Input: part model. Units: mm. Frame: model coordinates. Face numbers are marked on the shaded views. A direction names the side the tool comes from. Give positions to 0.01 mm unless a question says otherwise; leave off trailing zeros. Order: outer loops, then holes, each group sorted by start corner. A loop starts at its lowest first (then second) coordinate and runs counter-clockwise, first axis right, second up. Notation, with made-up numbers: M 40,69 L 72,69 A18 ccw 72,94 Z; hole C -27.5,89 d4. An arc over 180 degrees is marked long. Use a Markdown table: item, result.
from build123d import *

# Parameters (mm, degrees)
SKETCH_1_R      = 5.05
SKETCH_1_R_2    = 4.875
EXTRUDE_1_DEPTH = 10
FILLET_1_R      = 1


with BuildPart() as part:
    # 草图1 → 凸台-拉伸1 (new body)
    with BuildSketch(Plane.XY):
        with BuildLine():
            Line((100.75, 13), (39.610949593, 13))
            ThreePointArc((39.610949593, 13), (42.143955384, 14.911655633), (44.291298968, 17.248204611))
            ThreePointArc((44.291298968, 17.248204611), (43.91314903, 18.189421895), (43.515000291, 19.122355404))
            ThreePointArc((43.515000291, 19.122355404), (39.135260233, 19.155630081), (34.883671922, 18.103381529))
            ThreePointArc((34.883671922, 18.103381529), (34.03604328, 19.65071875), (33.119824259, 21.158455298))
            ThreePointArc((33.119824259, 21.158455298), (36.156892392, 24.314314506), (38.317945706, 28.123917996))
            ThreePointArc((38.317945706, 28.123917996), (37.709075956, 28.935191673), (37.083032847, 29.733287767))
            ThreePointArc((37.083032847, 29.733287767), (32.843916692, 28.631868497), (29.009539705, 26.515082418))
            ThreePointArc((29.009539705, 26.515082418), (27.790312967, 27.790312967), (26.515082418, 29.009539705))
            ThreePointArc((26.515082418, 29.009539705), (28.631868497, 32.843916692), (29.733287767, 37.083032847))
            ThreePointArc((29.733287767, 37.083032847), (28.935191673, 37.709075956), (28.123917996, 38.317945706))
            ThreePointArc((28.123917996, 38.317945706), (24.314314506, 36.156892392), (21.158455298, 33.119824259))
            ThreePointArc((21.158455298, 33.119824259), (19.65071875, 34.03604328), (18.103381529, 34.883671922))
            ThreePointArc((18.103381529, 34.883671922), (19.155630081, 39.135260233), (19.122355404, 43.515000291))
            ThreePointArc((19.122355404, 43.515000291), (18.189421895, 43.91314903), (17.248204611, 44.291298968))
            ThreePointArc((17.248204611, 44.291298968), (14.127731967, 41.217883822), (11.865457128, 37.46750481))
            ThreePointArc((11.865457128, 37.46750481), (10.171960525, 37.962273492), (8.457965105, 38.380539546))
            ThreePointArc((8.457965105, 38.380539546), (8.37396713, 42.759600464), (7.208266121, 46.981492378))
            ThreePointArc((7.208266121, 46.981492378), (6.204073074, 47.124613567), (5.197054586, 47.2462734))
            ThreePointArc((5.197054586, 47.2462734), (2.978367841, 43.469944586), (1.763847663, 39.261836826))
            ThreePointArc((1.763847663, 39.261836826), (0, 39.3014375), (-1.763847663, 39.261836826))
            ThreePointArc((-1.763847663, 39.261836826), (-2.978367841, 43.469944586), (-5.197054586, 47.2462734))
            ThreePointArc((-5.197054586, 47.2462734), (-6.204073074, 47.124613567), (-7.208266121, 46.981492378))
            ThreePointArc((-7.208266121, 46.981492378), (-8.37396713, 42.759600464), (-8.457965105, 38.380539546))
            ThreePointArc((-8.457965105, 38.380539546), (-10.171960525, 37.962273492), (-11.865457128, 37.46750481))
            ThreePointArc((-11.865457128, 37.46750481), (-14.127731967, 41.217883822), (-17.248204611, 44.291298968))
            ThreePointArc((-17.248204611, 44.291298968), (-18.189421895, 43.91314903), (-19.122355404, 43.515000291))
            ThreePointArc((-19.122355404, 43.515000291), (-19.155630081, 39.135260233), (-18.103381529, 34.883671922))
            ThreePointArc((-18.103381529, 34.883671922), (-19.65071875, 34.03604328), (-21.158455298, 33.119824259))
            ThreePointArc((-21.158455298, 33.119824259), (-24.314314506, 36.156892392), (-28.123917996, 38.317945706))
            ThreePointArc((-28.123917996, 38.317945706), (-28.935191673, 37.709075956), (-29.733287767, 37.083032847))
            ThreePointArc((-29.733287767, 37.083032847), (-28.631868497, 32.843916692), (-26.515082418, 29.009539705))
            ThreePointArc((-26.515082418, 29.009539705), (-27.790312967, 27.790312967), (-29.009539705, 26.515082418))
            ThreePointArc((-29.009539705, 26.515082418), (-32.843916692, 28.631868497), (-37.083032847, 29.733287767))
            ThreePointArc((-37.083032847, 29.733287767), (-37.709075956, 28.935191673), (-38.317945706, 28.123917996))
            ThreePointArc((-38.317945706, 28.123917996), (-36.156892392, 24.314314506), (-33.119824259, 21.158455298))
            ThreePointArc((-33.119824259, 21.158455298), (-34.03604328, 19.65071875), (-34.883671922, 18.103381529))
            ThreePointArc((-34.883671922, 18.103381529), (-39.135260233, 19.155630081), (-43.515000291, 19.122355404))
            ThreePointArc((-43.515000291, 19.122355404), (-43.91314903, 18.189421895), (-44.291298968, 17.248204611))
            ThreePointArc((-44.291298968, 17.248204611), (-41.217883822, 14.127731967), (-37.46750481, 11.865457128))
            ThreePointArc((-37.46750481, 11.865457128), (-37.962273492, 10.171960525), (-38.380539546, 8.457965105))
            ThreePointArc((-38.380539546, 8.457965105), (-42.759600464, 8.37396713), (-46.981492378, 7.208266121))
            ThreePointArc((-46.981492378, 7.208266121), (-47.124613567, 6.204073074), (-47.2462734, 5.197054586))
            ThreePointArc((-47.2462734, 5.197054586), (-43.469944586, 2.978367841), (-39.261836826, 1.763847663))
            ThreePointArc((-39.261836826, 1.763847663), (-39.3014375, 0), (-39.261836826, -1.763847663))
            ThreePointArc((-39.261836826, -1.763847663), (-43.469944586, -2.978367841), (-47.2462734, -5.197054586))
            ThreePointArc((-47.2462734, -5.197054586), (-47.124613567, -6.204073074), (-46.981492378, -7.208266121))
            ThreePointArc((-46.981492378, -7.208266121), (-42.759600464, -8.37396713), (-38.380539546, -8.457965105))
            ThreePointArc((-38.380539546, -8.457965105), (-37.962273492, -10.171960525), (-37.46750481, -11.865457128))
            ThreePointArc((-37.46750481, -11.865457128), (-41.217883822, -14.127731967), (-44.291298968, -17.248204611))
            ThreePointArc((-44.291298968, -17.248204611), (-43.91314903, -18.189421895), (-43.515000291, -19.122355404))
            ThreePointArc((-43.515000291, -19.122355404), (-39.135260233, -19.155630081), (-34.883671922, -18.103381529))
            ThreePointArc((-34.883671922, -18.103381529), (-34.03604328, -19.65071875), (-33.119824259, -21.158455298))
            ThreePointArc((-33.119824259, -21.158455298), (-36.156892392, -24.314314506), (-38.317945706, -28.123917996))
            ThreePointArc((-38.317945706, -28.123917996), (-37.709075956, -28.935191673), (-37.083032847, -29.733287767))
            ThreePointArc((-37.083032847, -29.733287767), (-32.843916692, -28.631868497), (-29.009539705, -26.515082418))
            ThreePointArc((-29.009539705, -26.515082418), (-27.790312967, -27.790312967), (-26.515082418, -29.009539705))
            ThreePointArc((-26.515082418, -29.009539705), (-28.631868497, -32.843916692), (-29.733287767, -37.083032847))
            ThreePointArc((-29.733287767, -37.083032847), (-28.935191673, -37.709075956), (-28.123917996, -38.317945706))
            ThreePointArc((-28.123917996, -38.317945706), (-24.314314506, -36.156892392), (-21.158455298, -33.119824259))
            ThreePointArc((-21.158455298, -33.119824259), (-19.65071875, -34.03604328), (-18.103381529, -34.883671922))
            ThreePointArc((-18.103381529, -34.883671922), (-19.155630081, -39.135260233), (-19.122355404, -43.515000291))
            ThreePointArc((-19.122355404, -43.515000291), (-18.189421895, -43.91314903), (-17.248204611, -44.291298968))
            ThreePointArc((-17.248204611, -44.291298968), (-14.127731967, -41.217883822), (-11.865457128, -37.46750481))
            ThreePointArc((-11.865457128, -37.46750481), (-10.171960525, -37.962273492), (-8.457965105, -38.380539546))
            ThreePointArc((-8.457965105, -38.380539546), (-8.37396713, -42.759600464), (-7.208266121, -46.981492378))
            ThreePointArc((-7.208266121, -46.981492378), (-6.204073074, -47.124613567), (-5.197054586, -47.2462734))
            ThreePointArc((-5.197054586, -47.2462734), (-2.978367841, -43.469944586), (-1.763847663, -39.261836826))
            ThreePointArc((-1.763847663, -39.261836826), (0, -39.3014375), (1.763847663, -39.261836826))
            ThreePointArc((1.763847663, -39.261836826), (2.978367841, -43.469944586), (5.197054586, -47.2462734))
            ThreePointArc((5.197054586, -47.2462734), (6.204073074, -47.124613567), (7.208266121, -46.981492378))
            ThreePointArc((7.208266121, -46.981492378), (8.37396713, -42.759600464), (8.457965105, -38.380539546))
            ThreePointArc((8.457965105, -38.380539546), (10.171960525, -37.962273492), (11.865457128, -37.46750481))
            ThreePointArc((11.865457128, -37.46750481), (14.127731967, -41.217883822), (17.248204611, -44.291298968))
            ThreePointArc((17.248204611, -44.291298968), (18.189421895, -43.91314903), (19.122355404, -43.515000291))
            ThreePointArc((19.122355404, -43.515000291), (19.155630081, -39.135260233), (18.103381529, -34.883671922))
            ThreePointArc((18.103381529, -34.883671922), (19.65071875, -34.03604328), (21.158455298, -33.119824259))
            ThreePointArc((21.158455298, -33.119824259), (24.314314506, -36.156892392), (28.123917996, -38.317945706))
            ThreePointArc((28.123917996, -38.317945706), (28.935191673, -37.709075956), (29.733287767, -37.083032847))
            ThreePointArc((29.733287767, -37.083032847), (28.631868497, -32.843916692), (26.515082418, -29.009539705))
            ThreePointArc((26.515082418, -29.009539705), (27.790312967, -27.790312967), (29.009539705, -26.515082418))
            ThreePointArc((29.009539705, -26.515082418), (32.843916692, -28.631868497), (37.083032847, -29.733287767))
            ThreePointArc((37.083032847, -29.733287767), (37.709075956, -28.935191673), (38.317945706, -28.123917996))
            ThreePointArc((38.317945706, -28.123917996), (36.156892392, -24.314314506), (33.119824259, -21.158455298))
            ThreePointArc((33.119824259, -21.158455298), (34.03604328, -19.65071875), (34.883671922, -18.103381529))
            ThreePointArc((34.883671922, -18.103381529), (39.135260233, -19.155630081), (43.515000291, -19.122355404))
            ThreePointArc((43.515000291, -19.122355404), (43.91314903, -18.189421895), (44.291298968, -17.248204611))
            ThreePointArc((44.291298968, -17.248204611), (42.143955384, -14.911655633), (39.610949593, -13))
            Line((39.610949593, -13), (100.75, -13))
            ThreePointArc((100.75, -13), (113.75, 0), (100.75, 13))
        make_face()
        with Locations((100.75, 0)):
            Circle(SKETCH_1_R, mode=Mode.SUBTRACT)
        Circle(SKETCH_1_R_2, mode=Mode.SUBTRACT)
    extrude(amount=EXTRUDE_1_DEPTH)

    # 圆角1
    fillet_1_edges = [part.edges().sort_by_distance(p)[0] for p in [
        (70.180474796, 13, 0),
        (113.75, 0, 0),
        (70.180474796, -13, 10),
        (113.75, 0, 10),
        (70.180474796, -13, 0),
        (70.180474796, 13, 10),
    ]]
    fillet(fillet_1_edges, radius=FILLET_1_R)


solid = part.part
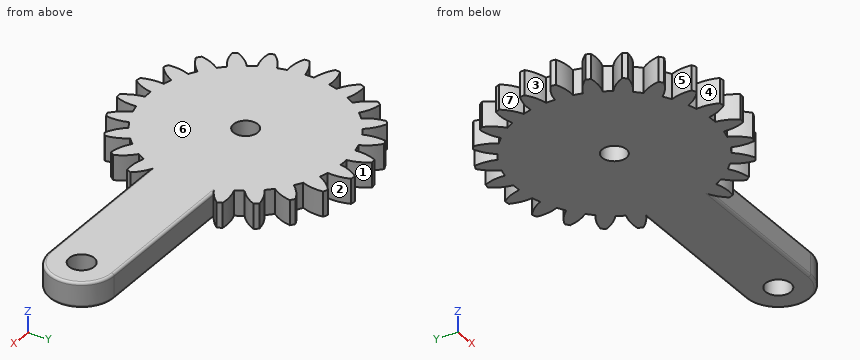
1) Cut plane C-C on x = 55. Return loops of the section in (y, z).
Response values:
| item | result |
|---|---|
| outline | M -13,1 A1 ccw -12,0 L 12,0 A1 ccw 13,1 L 13,9 A1 ccw 12,10 L -12,10 A1 ccw -13,9 Z |
2) Material intervals for line 1 (X direction, y = 0.5, z = 4.5); line 2 (Y direction, x = 100.75, z = 5.25); line 3 (X direction, y = -28, z = 7.25), sorted ascending. Write a range as from..to.
Response values:
| item | result |
|---|---|
| line 1 | x = -39.3..-4.85, 4.85..95.72, 105.78..113.74 |
| line 2 | y = -13..-5.05, 5.05..13 |
| line 3 | x = -38.27..-31.44, -27.58..27.58, 31.44..38.27 |
3) Cut plane B-B on y = 0. Return loops of the section in (x, z) (3 decimals).
Response values:
| item | result |
|---|---|
| outline | M -39.301,0 L -4.875,0 L -4.875,10 L -39.301,10 Z; M 4.875,0 L 95.7,0 L 95.7,10 L 4.875,10 Z; M 105.8,0 L 112.75,0 A1 ccw 113.75,1 L 113.75,9 A1 ccw 112.75,10 L 105.8,10 Z |
4) Cut plane A-A on x = 0. Return loops of the section in (y, z) (3 decimals), and give its area (3 significant figures).
Response values:
| item | result |
|---|---|
| outline | M -39.301,0 L -4.875,0 L -4.875,10 L -39.301,10 Z; M 4.875,0 L 39.301,0 L 39.301,10 L 4.875,10 Z |
| area | 689 mm² |
5) First-contact query: pin 1 Ø2.5 at (x, z) = (70.5, 4) entering from -Y; pin 2 Ø1 at (x, z) = (62, 6.5) entering from +Y; pin 3 Ø1 at (y, z) = (-23.5, 3) entering from +X. Flat tips, straight axial feed; report the tip coordinate or a pass-through.
Response values:
| item | result |
|---|---|
| pin 1 | stops at y = -13 |
| pin 2 | stops at y = 13 |
| pin 3 | stops at x = 35.92 |
6) Mould query, pull axis X, two halves, no side actions, for the marked faces 4, 5, 6 and 7. Classes: released by +X, released by -X, zero draft, split by the parting line, or undercut.
Response values:
| item | result |
|---|---|
| face 4 | undercut |
| face 5 | undercut |
| face 6 | zero draft |
| face 7 | released by -X |
7) Cut plane D-D on z = 5.75. State how many separate pieces and enclosed holes the cut face has, and give its area (3 significant figures).
Response values:
| item | result |
|---|---|
| separate pieces | 1 |
| enclosed holes | 2 |
| area | 7,510 mm² |
8) Reachability of the marked faces 1, 2 and 3 from +Z, -Z, +X, -X, +Y, -Y: full face, straight path, thin tool, end or side. Return the list, or none.
Response values:
| item | result |
|---|---|
| face 1 | +Z, -Z, +Y |
| face 2 | +Z, -Z |
| face 3 | +Z, -Z, -X |
